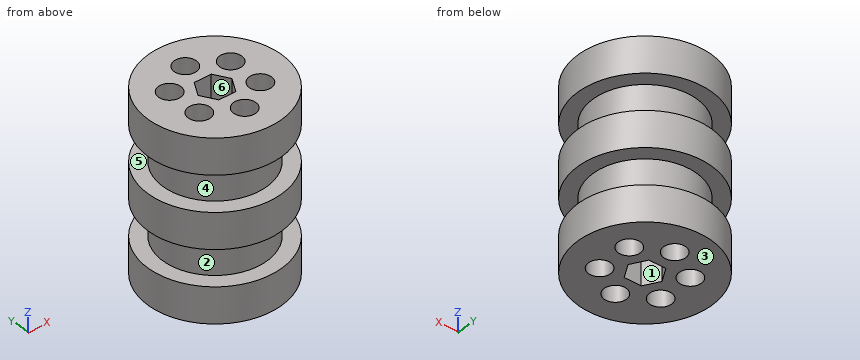
Autodesk Inventor part; units mm, degrees
ref_plane "Work Plane5" through (-2.7496, 1.5875, -11.43) normal (0, 0, 1) x (1, 0, 0)
ref_plane "YZ Plane" through (0, 0, 0) normal (1, 0, 0) x (0, 1, 0)
ref_plane "XZ Plane" through (0, 0, 0) normal (0, 1, 0) x (-1, 0, 0)
sketch "Sketch1" plane through (0, 0, 0) normal (0, 0, 1) x (1, 0, 0)
  line L0 (-1.8331, 3.175) -> (1.8331, 3.175)
  line L1 (1.8331, 3.175) -> (3.6662, 0)
  line L2 (3.6662, 0) -> (1.8331, -3.175)
  line L3 (1.8331, -3.175) -> (-1.8331, -3.175)
  line L4 (-1.8331, -3.175) -> (-3.6662, 0)
  line L5 (-3.6662, 0) -> (-1.8331, 3.175)
  circle A0 centre (0, 0) radius 14.2875
  dimension "d1" = 6.35
  dimension "d4" = 28.575
extrude "Extrusion1" add sketch "Sketch1" along normal mid plane 38.1
ref_plane "Work Plane5" through (-2.7496, 1.5875, -11.43) normal (0, 0, 1) x (1, 0, 0)
ref_plane "Work Plane4" through (-2.7496, 1.5875, -3.81) normal (0, 0, 1) x (1, 0, 0)
sketch "Sketch2" plane through (-2.7496, 1.5875, 11.43) normal (0, 0, 1) x (1, 0, 0)
  circle A0 centre (2.7496, -1.5875) radius 11.1125
  circle A1 centre (2.7496, -1.5875) radius 14.2875
  dimension "d9" = 22.225
extrude "Extrusion2" cut sketch "Sketch2" against normal blind 7.62
sketch "Sketch3" plane through (-2.7496, 1.5875, -3.81) normal (0, 0, 1) x (1, 0, 0)
  circle A0 centre (2.7496, -1.5875) radius 14.2875
  circle A1 centre (2.7496, -1.5875) radius 11.1125
  point P0 (2.7351, -1.6125)
sketch "Sketch4" plane through (0, 0, -19.05) normal (0, 0, -1) x (-1, 0, 0)
  circle A0 centre (0, 0) radius 14.2875
  point P0 (0, 7.62)
  point P1 (-6.5991, 3.81)
  point P2 (-6.5991, -3.81)
  point P3 (0, -7.62)
  point P4 (6.5991, -3.81)
  point P5 (6.5991, 3.81)
  dimension "d15" = 7.62
  dimension "d18" = 360
hole "Hole1" at (0, 7.62, -19.05) at (6.5991, 3.81, -19.05) at (6.5991, -3.81, -19.05) at (0, -7.62, -19.05) at (-6.5991, -3.81, -19.05) at (-6.5991, 3.81, -19.05) direction (0, 0, 1) diameter 4.7625 end through all
extrude "Extrusion4" cut sketch "Sketch3" against normal blind 7.62
ref_plane "Work Plane1" through (-2.7496, 1.5875, 19.05) normal (0, 0, 1) x (1, 0, 0)
ref_plane "Work Plane2" through (-2.7496, 1.5875, 11.43) normal (0, 0, 1) x (1, 0, 0)
ref_plane "Work Plane3" through (-2.7496, 1.5875, 3.81) normal (0, 0, 1) x (1, 0, 0)
properties part number "WheelHub" material "Aluminum-6061"
Source: CAD feature listing. Evaluate the final solid. Frame: model axes, mm. Face numbers are marked on the shaded views. A direction names the side the tool comes from. Coordinates: 2 decimals unless noted, no trailing zeros. Loops run counter-clockwise (first coordinate to the right, second up) from the corner with the lowest first, then second, coordinate; pieces in that order, holes last. Notation, with made-up numbers: M -17.75,15.5 L 21.25,15.5 A19 cw 21.25,48.5 Z; hole C -22,-30 d7. An arc over 180 degrees is marked long. Use CSV: the item, a comma, the result in double quotes.
(1) Line query: line 1 (Y direction, x = 0, z = 1.5) (1 decimal); line 2 (Z direction, x = 11.75, y = -8); line 3 (X direction, y = -2.25, z = 0). Output: solid intervals per line, ascending. Write a range as [from, to].
Answers follow:
line 1,"[-14.3, -10], [-5.2, -3.2], [3.2, 5.2], [10, 14.3]"
line 2,"[-19.05, -11.43], [-3.81, 3.81], [11.43, 19.05]"
line 3,"[-14.11, -8.4], [-4.8, -2.37], [2.37, 4.8], [8.4, 14.11]"
(2) Draft query along X for the marked faces 4, 5 and 6. Return one class per face: pulls with the +X half, pulls with the -X half, needs draft (parallel to the pull), parting line crosses it, or undercut.
Answers follow:
face 4,"parting line crosses it"
face 5,"needs draft"
face 6,"undercut"
(3) Cut plane A-A on x = 0. Give the number of separate pieces and of enclosed holes in the cut face, and give its area (3 significant figures).
Answers follow:
separate pieces,"4"
enclosed holes,"0"
area,"387 mm²"
(4) Cut plane D-D on y = 8. Return loops of the section in (x, z).
Answers follow:
outline,"M -11.84,-19.05 L -2.35,-19.05 L -2.35,19.05 L -11.84,19.05 L -11.84,11.43 L -7.71,11.43 L -7.71,3.81 L -11.84,3.81 L -11.84,-3.81 L -7.71,-3.81 L -7.71,-11.43 L -11.84,-11.43 Z; M 2.35,-19.05 L 11.84,-19.05 L 11.84,-11.43 L 7.71,-11.43 L 7.71,-3.81 L 11.84,-3.81 L 11.84,3.81 L 7.71,3.81 L 7.71,11.43 L 11.84,11.43 L 11.84,19.05 L 2.35,19.05 Z"
(5) Reachability of the marked faces 1, 2 and 3 from +Z, -Z, +X, -X, +Y, -Y: full face, straight path, thin tool, end or side. Return the list, or none.
Answers follow:
face 1,"+Z, -Z"
face 2,"none"
face 3,"-Z, +X, -X, +Y, -Y"
(6) Cut plane C-C on x = -5.75. Return loops of the section in (y, z).
Answers follow:
outline,"M -13.08,-19.05 L -6.03,-19.05 L -6.03,19.05 L -13.08,19.05 L -13.08,11.43 L -9.51,11.43 L -9.51,3.81 L -13.08,3.81 L -13.08,-3.81 L -9.51,-3.81 L -9.51,-11.43 L -13.08,-11.43 Z; M -1.59,-19.05 L 1.59,-19.05 L 1.59,19.05 L -1.59,19.05 Z; M 6.03,-19.05 L 13.08,-19.05 L 13.08,-11.43 L 9.51,-11.43 L 9.51,-3.81 L 13.08,-3.81 L 13.08,3.81 L 9.51,3.81 L 9.51,11.43 L 13.08,11.43 L 13.08,19.05 L 6.03,19.05 Z"
(7) Cut plane B-B on z = -5. Return loops of the section in (x, y) (1 decimal), and give its area (3 significant figures).
Answers follow:
outline,"C 0,0 d22.2; hole C -6.6,-3.8 d4.8; hole C -6.6,3.8 d4.8; hole M -3.7,0 L -1.8,-3.2 L 1.8,-3.2 L 3.7,0 L 1.8,3.2 L -1.8,3.2 Z; hole C 0,-7.6 d4.8; hole C 0,7.6 d4.8; hole C 6.6,-3.8 d4.8; hole C 6.6,3.8 d4.8"
area,"246 mm²"
(8) Contact query for flat-ended pins moving along their axis: pin 1 (8 mm diameter, centred on y = -5, z = -11, fed in from -X); pin 2 (4 mm diameter, centred on x = -3.5, z = 2, fed in from -Y); pin 3 (3 mm diameter, centred on x = -0.5, z = -7.5, fed in from -Y). Output: stop coordinate, or through.
Answers follow:
pin 1,"x = -14.25"
pin 2,"y = -14.21"
pin 3,"y = -11.11"
